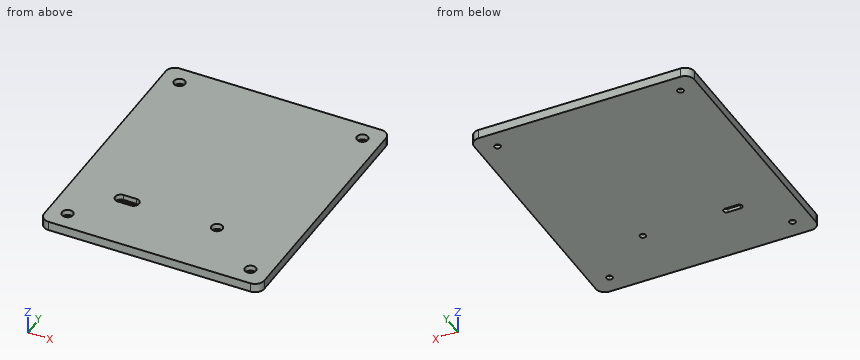
```python
from build123d import *

# Parameters (mm, degrees)
SKETCH1_W           = 120
SKETCH1_H           = 140
SKETCH1_R           = 1.65
BOSS_EXTRUDE1_DEPTH = 5
FILLET3_R           = 5
SKETCH3_R           = 1.6
CUT_EXTRUDE3_DEPTH  = 5
SKETCH2_R           = 3
SKETCH2_R_2         = 1.6
CUT_EXTRUDE1_DEPTH  = 3


with BuildPart() as part:
    # Sketch1 → Boss-Extrude1 (new body)
    with BuildSketch(Plane.XY):
        Rectangle(SKETCH1_W, SKETCH1_H)
        with Locations((-49.85, -59.85)):
            Circle(SKETCH1_R, mode=Mode.SUBTRACT)
        with Locations((49.85, -59.85)):
            Circle(SKETCH1_R, mode=Mode.SUBTRACT)
        with Locations((49.85, 59.85)):
            Circle(SKETCH1_R, mode=Mode.SUBTRACT)
        with Locations((-49.85, 59.85)):
            Circle(SKETCH1_R, mode=Mode.SUBTRACT)
    extrude(amount=BOSS_EXTRUDE1_DEPTH)

    # Fillet3
    fillet3_edges = [part.edges().sort_by_distance(p)[0] for p in [
        (60, -70, 2.5),
        (-60, -70, 2.5),
        (-60, 70, 2.5),
        (60, 70, 2.5),
    ]]
    fillet(fillet3_edges, radius=FILLET3_R)

    # Sketch3 → Cut-Extrude3 (cut)
    with BuildSketch(Plane.XY.offset(5)):
        with Locations((20, -37)):
            Circle(SKETCH3_R)
        with BuildLine():
            Line((-32.5, -35.4), (-25.5, -35.4))
            ThreePointArc((-25.5, -35.4), (-23.9, -37), (-25.5, -38.6))
            Line((-25.5, -38.6), (-32.5, -38.6))
            ThreePointArc((-32.5, -38.6), (-34.1, -37), (-32.5, -35.4))
        make_face()
    extrude(amount=-CUT_EXTRUDE3_DEPTH, mode=Mode.SUBTRACT)

    # Sketch2 → Cut-Extrude1 (cut)
    # profile 1 of 6: a face of its own
    with BuildSketch(Plane.XY.offset(5)):
        with Locations((-49.85, 59.85)):
            Circle(SKETCH2_R)
    # profile 2 of 6: a face of its own
    with BuildSketch(Plane.XY.offset(5)):
        with Locations((49.85, 59.85)):
            Circle(SKETCH2_R)
    # profile 3 of 6: a face of its own
    with BuildSketch(Plane.XY.offset(5)):
        with Locations((49.85, -59.85)):
            Circle(SKETCH2_R)
    # profile 4 of 6: a face of its own
    with BuildSketch(Plane.XY.offset(5)):
        with Locations((-49.85, -59.85)):
            Circle(SKETCH2_R)
    # profile 5 of 6: a face of its own
    with BuildSketch(Plane.XY.offset(5)):
        with Locations((20, -37)):
            Circle(SKETCH2_R)
        with Locations((20, -37)):
            Circle(SKETCH2_R_2, mode=Mode.SUBTRACT)
    # profile 6 of 6: a face of its own
    with BuildSketch(Plane.XY.offset(5)):
        with BuildLine():
            Line((-32.5, -34), (-25.5, -34))
            ThreePointArc((-25.5, -34), (-22.5, -37), (-25.5, -40))
            Line((-25.5, -40), (-32.5, -40))
            ThreePointArc((-32.5, -40), (-35.5, -37), (-32.5, -34))
        make_face()
        with BuildLine():
            Line((-32.5, -35.4), (-25.5, -35.4))
            ThreePointArc((-25.5, -35.4), (-23.9, -37), (-25.5, -38.6))
            Line((-25.5, -38.6), (-32.5, -38.6))
            ThreePointArc((-32.5, -38.6), (-34.1, -37), (-32.5, -35.4))
        make_face(mode=Mode.SUBTRACT)
    extrude(amount=-CUT_EXTRUDE1_DEPTH, mode=Mode.SUBTRACT)


solid = part.part
```
The listing builds one solid part. Answer for the finished solid, in the listing's coordinates (mm). Coordinates: 2 decimals unless noted, no trailing zeros. Write each loop counter-clockwise with the first axis right and the second up, starting at its lowest first coordinate (ties: lowest second). Pieces come first, ordered by that corner, then holes.
Q1. Given P1, Ø8, axis at x = 49.85, y = 59.85, coming from the +Z side; P2, Ø3, axis at x = 49.85, y = -59.85, coming from the -Z side; P3, Ø5, axis at x = 20, y = -37, coming from the +Z side, each flat-ended and moving along its own axis, determine where each tip first touches the part or whether it passes through.
Returned:
P1: stops at z = 5
P2: passes through
P3: stops at z = 2
Q2. Find the intervals of material crossed by line 1 along Y through (x, z) = (-49.85, 2.75); line 2 along X through (y, z) = (-59.85, 1); line 3 along Y through (x, z) = (-51, 4.05), in increasing order.
Returned:
line 1: y = -70 to -62.85, -56.85 to 56.85, 62.85 to 70
line 2: x = -60 to -51.5, -48.2 to 48.2, 51.5 to 60
line 3: y = -70 to -62.62, -57.08 to 57.08, 62.62 to 70
Q3. Section A-A, the plane y = 59.85 is taken. Write down the section's boundary in (x, z).
Returned:
outline: (-60, 0) - (-51.5, 0) - (-51.5, 2) - (-52.85, 2) - (-52.85, 5) - (-60, 5) - close; (-48.2, 0) - (48.2, 0) - (48.2, 2) - (46.85, 2) - (46.85, 5) - (-46.85, 5) - (-46.85, 2) - (-48.2, 2) - close; (51.5, 0) - (60, 0) - (60, 5) - (52.85, 5) - (52.85, 2) - (51.5, 2) - close
Q4. Section B-B, the plane x = 49.85 is taken. Write down the section's boundary in (y, z), then the cut area to 3 significant figures.
Returned:
outline: (-70, 0) - (-61.5, 0) - (-61.5, 2) - (-62.85, 2) - (-62.85, 5) - (-70, 5) - close; (-58.2, 0) - (58.2, 0) - (58.2, 2) - (56.85, 2) - (56.85, 5) - (-56.85, 5) - (-56.85, 2) - (-58.2, 2) - close; (61.5, 0) - (70, 0) - (70, 5) - (62.85, 5) - (62.85, 2) - (61.5, 2) - close
area: 651 mm2
Q5. Section C-C, the plane x = 20 is taken. Write down the section's boundary in (y, z), then the cut area to 3 significant figures.
Returned:
outline: (-70, 0) - (-38.6, 0) - (-38.6, 2) - (-40, 2) - (-40, 5) - (-70, 5) - close; (-35.4, 0) - (70, 0) - (70, 5) - (-34, 5) - (-34, 2) - (-35.4, 2) - close
area: 676 mm2
